Design review of the part built by this model. Coordinates are the model's own, in mm. Face numbers are marked on the shaded views. A direction names the side the tool comes from. Give positions to 0.01 mm unless a question says otherwise; leave off trailing zeros. Loops run counter-clockwise (first coordinate to the right, second up) from the corner with the lowest first, then second, coordinate; pieces in that order, holes last. Notation, with made-up numbers: (-35, -15) -> (-10, -15) arc R11 cw to (-10, 5) -> close; hole circle Ø6 at (-7.5, 1). An arc over 180 degrees is marked (long way). Use a Markdown table: item, result. Add a question column.
1. For pin 1 Ø1 at (x, z) = (-231.5, -24) entering from -Y; pin 2 Ø5 at (x, z) = (-244.5, -4) entering from +Y; pin 3 Ø9 at (x, z) = (-275, -20) entering from -Y; pin 4 Ø4 at (x, y) = (-263, 23.5) entering from +Z, all flat-tipped, find the tip position at first contact; note any pin that passes through.
2. Add section C-C (y = 24.5). State the section outline as (x, z) points.
3. Draft analysis for pull direction X (two halves, no side actions). For the marked faces 4, 5 and 6, state which applies: pulls with the +X half, pulls with the -X half, needs draft (parallel to the pull), parting line crosses it, or undercut.
4. For the marked faces 1, 2 and 3, list the 3-axis set-ups (+Z, -Z, +X, -X, +Y, -Y) from which the entire face can be reached by the end or side of a thin tool; tool diameter is ignored.
5. Add section A-A (z = -15). State the section outline as (x, y) points.
6. Add section D-D (z = -1.75). State the section outline as (x, y) points, and give its area (3 significant figures).
7. Add section B-B (x = -259). State the section outline as (y, z) points, and give its area (3 significant figures).
8. To check wall thickness, follow line 1 (X direction, y = 1, z = -13.5); line 2 (Y direction, x = -251.5, z = -16.25); line 3 (Y direction, x = -294, z = -16.5). State the ranges of each line that lie inside material, in increasing order.
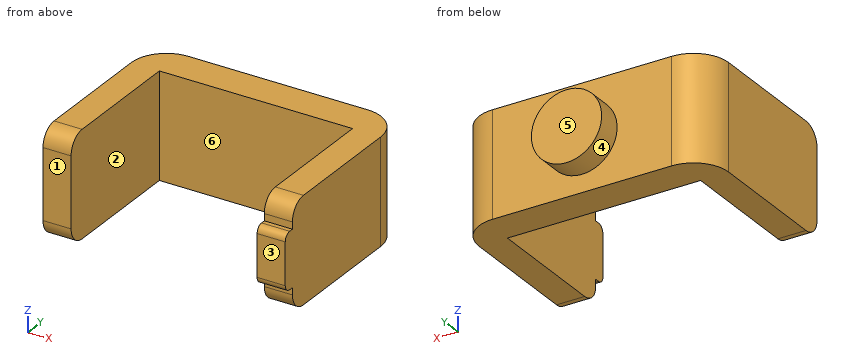
```python
from build123d import *

# Parameters (mm, degrees)
BOSS_EXTRUDE1_DEPTH = 30
SKETCH2_R           = 10
BOSS_EXTRUDE2_DEPTH = 7
FILLET1_R           = 5
FILLET2_R           = 10
SKETCH3_W           = 8
SKETCH3_H           = 16
BOSS_EXTRUDE3_DEPTH = 3.25
FILLET3_R           = 2


with BuildPart() as part:
    # Sketch1 → Boss-Extrude1 (new body)
    with BuildSketch(Plane.XY):
        Polygon((-289.346773142, -20.703646913), (-289.346773142, 19.296353087), (-234.346773142, 19.296353087), (-234.346773142, -20.703646913), (-226.346773142, -20.703646913), (-226.346773142, 29.296353087), (-297.346773142, 29.296353087), (-297.346773142, -20.703646913), align=None)
    extrude(amount=-BOSS_EXTRUDE1_DEPTH)

    # Sketch2 → Boss-Extrude2 (add)
    with BuildSketch(Plane(origin=(0, 29.296353087, 0), x_dir=(1, 0, 0), z_dir=(0, 1, 0))):
        with Locations((-261.846773142, 15)):
            Circle(SKETCH2_R)
    extrude(amount=BOSS_EXTRUDE2_DEPTH)

    # Fillet1
    fillet1_edges = [part.edges().sort_by_distance(p)[0] for p in [
        (-293.346773142, -20.703646913, 0),
        (-293.346773142, -20.703646913, -30),
        (-230.346773142, -20.703646913, 0),
        (-230.346773142, -20.703646913, -30),
    ]]
    fillet(fillet1_edges, radius=FILLET1_R)

    # Fillet2
    fillet2_edges = [part.edges().sort_by_distance(p)[0] for p in [
        (-297.346773142, 29.296353087, -15),
        (-226.346773142, 29.296353087, -15),
    ]]
    fillet(fillet2_edges, radius=FILLET2_R)

    # Sketch3 → Boss-Extrude3 (add)
    with BuildSketch(Plane.XZ.offset(20.703646913)):
        with Locations((-230.346773142, -15)):
            Rectangle(SKETCH3_W, SKETCH3_H)
    extrude(amount=BOSS_EXTRUDE3_DEPTH)

    # Fillet3
    fillet3_edges = [part.edges().sort_by_distance(p)[0] for p in [
        (-230.346773142, -23.953646913, -7),
        (-230.346773142, -23.953646913, -23),
    ]]
    fillet(fillet3_edges, radius=FILLET3_R)


solid = part.part
```
Taken from the geometry:
| question | item | result |
|---|---|---|
| 1 | pin 1 | stops at y = -20.7 |
| 1 | pin 2 | stops at y = 29.3 |
| 1 | pin 3 | stops at y = 19.3 |
| 1 | pin 4 | stops at z = 0 |
| 2 | outline | (-295.89, -30) -> (-227.81, -30) -> (-227.81, 0) -> (-295.89, 0) -> close |
| 3 | face 4 | parting line crosses it |
| 3 | face 5 | needs draft |
| 3 | face 6 | undercut |
| 4 | face 1 | +Z, -Z, -X, -Y |
| 4 | face 2 | +Z, -Z, -Y |
| 4 | face 3 | +Z, -Z, +X, -X, -Y |
| 5 | outline | (-297.35, -20.7) -> (-289.35, -20.7) -> (-289.35, 19.3) -> (-234.35, 19.3) -> (-234.35, -23.95) -> (-226.35, -23.95) -> (-226.35, 19.3) arc R10 ccw to (-236.35, 29.3) -> (-251.85, 29.3) -> (-251.85, 36.3) -> (-271.85, 36.3) -> (-271.85, 29.3) -> (-287.35, 29.3) arc R10 ccw to (-297.35, 19.3) -> close |
| 6 | outline | (-297.35, -19.5) -> (-289.35, -19.5) -> (-289.35, 19.3) -> (-234.35, 19.3) -> (-234.35, -19.5) -> (-226.35, -19.5) -> (-226.35, 19.3) arc R10 ccw to (-236.35, 29.3) -> (-287.35, 29.3) arc R10 ccw to (-297.35, 19.3) -> close |
| 6 | area | 1,290 mm^2 |
| 7 | outline | (19.3, -30) -> (29.3, -30) -> (29.3, -24.59) -> (36.3, -24.59) -> (36.3, -5.41) -> (29.3, -5.41) -> (29.3, 0) -> (19.3, 0) -> close |
| 7 | area | 434 mm^2 |
| 8 | line 1 | x = -297.35 to -289.35, -234.35 to -226.35 |
| 8 | line 2 | y = 19.3 to 29.3 |
| 8 | line 3 | y = -20.7 to 26.76 |
